Read the model definition and answer for the solid it produces. Units are mm, in the model's axes. Face numbers are marked on the shaded views. A direction names the side the tool comes from. Give positions to 0.01 mm unless a question says otherwise; leave off trailing zeros. Order: outer loops, then holes, each group sorted by start corner. A loop starts at its lowest first (then second) coordinate and runs counter-clockwise, first axis right, second up. Notation, with made-up numbers: (51, -28.75) - (70, -28.75) arc R13 cw to (70, -12.75) - close; hole circle Ø11 at (21, -7). An arc over 180 degrees is marked (long way). Answer as CSV lines item,"result". Start each with the question number.
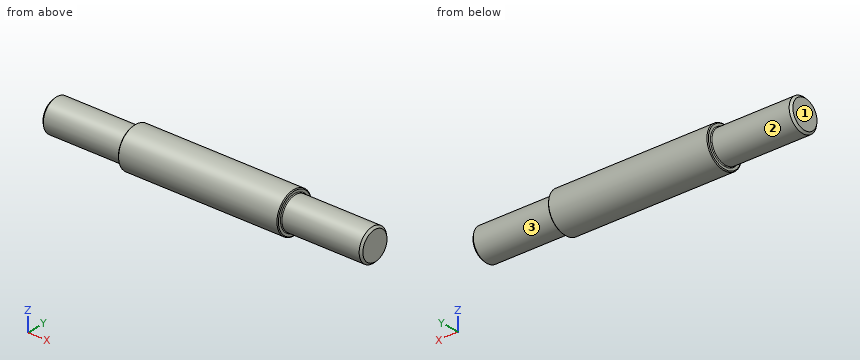
from build123d import *

# Parameters (mm, degrees)
CHAMFER1_SIZE = 0.2
CHAMFER2_SIZE = 0.2
CHAMFER3_SIZE = 0.5
CHAMFER4_SIZE = 0.5
FILLET1_R     = 0.2
FILLET2_R     = 0.2


with BuildPart() as part:
    # Sketch1 → Revolve1 (revolve)
    with BuildSketch(Plane.XY, mode=Mode.PRIVATE) as revolve1_sk:
        Polygon((0, 0), (80, 0), (80, 4), (60, 4), (60, 5), (20, 5), (20, 4), (0, 4), align=None)
    revolve(revolve1_sk.sketch.rotate(Axis((0, 0, 0), (1, 0, 0)), 90), axis=Axis((0, 0, 0), (1, 0, 0)))

    # Chamfer1
    chamfer1_edges = [part.edges().sort_by_distance(p)[0] for p in [
        (60, 0, -5),
    ]]
    chamfer(chamfer1_edges, length=CHAMFER1_SIZE)

    # Chamfer2
    chamfer2_edges = [part.edges().sort_by_distance(p)[0] for p in [
        (20, 0, -5),
    ]]
    chamfer(chamfer2_edges, length=CHAMFER2_SIZE)

    # Chamfer3
    chamfer3_edges = [part.edges().sort_by_distance(p)[0] for p in [
        (0, 0, -4),
    ]]
    chamfer(chamfer3_edges, length=CHAMFER3_SIZE)

    # Chamfer4
    chamfer4_edges = [part.edges().sort_by_distance(p)[0] for p in [
        (80, 0, -4),
    ]]
    chamfer(chamfer4_edges, length=CHAMFER4_SIZE)

    # Fillet1
    fillet1_edges = [part.edges().sort_by_distance(p)[0] for p in [
        (20, 0, -4),
    ]]
    fillet(fillet1_edges, radius=FILLET1_R)

    # Fillet2
    fillet2_edges = [part.edges().sort_by_distance(p)[0] for p in [
        (60, 0, -4),
    ]]
    fillet(fillet2_edges, radius=FILLET2_R)


solid = part.part
(1) Section C-C, the plane x = 30 is taken. Write down the section's boundary in (y, z), and give its area (3 significant figures).
(2) Which of the six approach directions +Z, -Z, +X, -X, +Y, -Y give full straight-line access (tool end or side, diameter ignored) to the marked faces 1, 2 and 3?
(3) Section A-A, the plane y = 0 is taken. Write down the section's boundary in (x, z).
(4) Straight lines are drawn through the part: line 1 (Y direction, x = 13, z = 0.25); line 2 (Y direction, x = 23.5, z = 0.25); line 3 (X direction, y = 1, z = 4). For each, find the intervals that lie inside material, in ascending order. Write a range as [from, to].
(5) Flat-ended cylindrical pins translate along their axes: pin 1 Ø5 at (y, z) = (-1.5, -2) entering from -X; pin 2 Ø1.5 at (x, z) = (52, -1.5) entering from +Y; pin 3 Ø6 at (x, z) = (60.5, 3.5) entering from +Y. Find the tip coordinate at first contact, or state that the pin passes through.
(6) Section D-D, the plane x = 74 is taken. Write down the section's boundary in (y, z), and give its area (3 significant figures).
Checks:
1,outline,"circle Ø10 at (0, 0)"
1,area,"78.5 mm²"
2,face 1,"+Z, -Z, -X, +Y, -Y"
2,face 2,"-X"
2,face 3,"+X"
3,outline,"(0, -3.5) - (0.5, -4) - (19.8, -4) arc R0.2 cw to (20, -4.2) - (20, -4.8) - (20.2, -5) - (59.8, -5) - (60, -4.8) - (60, -4.2) arc R0.2 cw to (60.2, -4) - (79.5, -4) - (80, -3.5) - (80, 3.5) - (79.5, 4) - (60.2, 4) arc R0.2 cw to (60, 4.2) - (60, 4.8) - (59.8, 5) - (20.2, 5) - (20, 4.8) - (20, 4.2) arc R0.2 cw to (19.8, 4) - (0.5, 4) - (0, 3.5) - close"
4,line 1,"y = [-3.99, 3.99]"
4,line 2,"y = [-4.99, 4.99]"
4,line 3,"x = [19.98, 60.02]"
5,pin 1,"stops at x = 0"
5,pin 2,"stops at y = 4.94"
5,pin 3,"stops at y = 4.97"
6,outline,"circle Ø8 at (0, 0)"
6,area,"50.3 mm²"
